```python
from build123d import *

# Parameters (mm, degrees)
SKETCH3_R           = 4.25
SKETCH3_R_2         = 3.75
BOSS_EXTRUDE1_DEPTH = 20
SKETCH21_R          = 10
BOSS_EXTRUDE2_DEPTH = 1
SKETCH29_R          = 1.75
CUT_EXTRUDE6_DEPTH  = 8.3
BOSS_EXTRUDE5_START = 1
SKETCH33_R          = 10
BOSS_EXTRUDE5_DEPTH = 1
SKETCH35_R          = 3.75
CUT_EXTRUDE8_DEPTH  = 27.153393661


with BuildPart() as part:
    # Sketch3 → Boss-Extrude1 (new body)
    with BuildSketch(Plane(origin=(0, 0, 0), x_dir=(1, 0, 0), z_dir=(0, 1, 0))):
        with Locations(Location((0, 0, 0), (0, 0, 270))):
            Circle(SKETCH3_R)
        with Locations(Location((0, 0, 0), (0, 0, 270))):
            Circle(SKETCH3_R_2, mode=Mode.SUBTRACT)
    extrude(amount=BOSS_EXTRUDE1_DEPTH)

    # Sketch21 → Boss-Extrude2 (add)
    with BuildSketch(Plane(origin=(0, 20, 0), x_dir=(1, 0, 0), z_dir=(0, 1, 0))):
        with Locations(Location((0, 0, 0), (0, 0, 270))):
            Circle(SKETCH21_R)
    extrude(amount=BOSS_EXTRUDE2_DEPTH)

    # Sketch29 → Cut-Extrude6 (cut)
    with BuildSketch(Plane(origin=(0, 21, 0), x_dir=(1, 0, 0), z_dir=(0, 1, 0))):
        with Locations(Location((0, 0, 0), (0, 0, 270))):
            Circle(SKETCH29_R)
    extrude(amount=-CUT_EXTRUDE6_DEPTH, mode=Mode.SUBTRACT)

    # Sketch33 → Boss-Extrude5 (add)
    with BuildSketch(Plane.XZ.offset(BOSS_EXTRUDE5_START)):
        with Locations(Location((0, 0, 0), (0, 0, 90))):
            Circle(SKETCH33_R)
    extrude(amount=-BOSS_EXTRUDE5_DEPTH)

    # Sketch35 → Cut-Extrude8 (cut, through all)
    with BuildSketch(Plane.XZ.offset(1)):
        with Locations(Location((0, 0, 0), (0, 0, 270))):
            Circle(SKETCH35_R)
    extrude(amount=-CUT_EXTRUDE8_DEPTH, mode=Mode.SUBTRACT)


solid = part.part
```
Read the model definition and answer for the solid it produces. Units are mm, in the model's axes. A direction names the side the tool comes from. Round coordinates to 2 decimals unless told otherwise and drop trailing zeros. Write each loop counter-clockwise with the first axis right and the second up, starting at its lowest first coordinate (ties: lowest second). Pieces come first, ordered by that corner, then holes. Notation, with made-up numbers: (16, 55.25) - (42, 55.25) arc R19 ccw to (42, 66.25) - close; hole circle Ø10 at (49, 32.25). An arc over 180 degrees is marked (long way). One line per item, written item: value.
Q1. Find section B-B (x = 2). Determine the outline of the cut face in (y, z), and give its area (3 significant figures).
The answers:
outline: (-1, -9.8) - (0, -9.8) - (0, -3.75) - (20, -3.75) - (20, -9.8) - (21, -9.8) - (21, -3.17) - (-1, -3.17) - close; (-1, 3.17) - (21, 3.17) - (21, 9.8) - (20, 9.8) - (20, 3.75) - (0, 3.75) - (0, 9.8) - (-1, 9.8) - close
area: 49.6 mm2
Q2. Each of these flat-tipped pins is pushed along its axis until it touches: P1, Ø10, axis at x = 5, y = 7.5, coming from the +Z side; P2, Ø6, axis at x = 0, z = 0, coming from the +Y side; P3, Ø1.5, axis at x = 2, y = 1.5, coming from the -Z side; P4, Ø2, axis at x = 1.5, y = 8.5, coming from the -Z side. Where does it stop, or does it pass through?
The answers:
P1: stops at z = 4.25
P2: passes through
P3: stops at z = -4.06
P4: stops at z = -4.22
Q3. Find section D-D (x = 7.75). Determine the outline of the cut face in (y, z), and give its area (3 significant figures).
The answers:
outline: (-1, -6.32) - (0, -6.32) - (0, 6.32) - (-1, 6.32) - close; (20, -6.32) - (21, -6.32) - (21, 6.32) - (20, 6.32) - close
area: 25.3 mm2
Q4. Find section A-A (z = 0). Determine the outline of the cut face in (x, y).
The answers:
outline: (-10, -1) - (-3.75, -1) - (-3.75, 21) - (-10, 21) - (-10, 20) - (-4.25, 20) - (-4.25, 0) - (-10, 0) - close; (3.75, -1) - (10, -1) - (10, 0) - (4.25, 0) - (4.25, 20) - (10, 20) - (10, 21) - (3.75, 21) - close
Q5. Find section C-C (y = 4.5). Determine the outline of the cut face in (x, z).
The answers:
outline: circle Ø8.5 at (0, 0); hole circle Ø7.5 at (0, 0)
Q6. For a pull along X with two mould halves and no side action, classify faces 1 (the flat face through (0, -1, 4)), 2 (the cylindrical face through (0.165, 9.846, 3.746)), 3 (the cylindrical face through (4.214, 9.86, -0.553)) as pulls with the +X half, pulls with the -X half, needs draft (parallel to the pull), parting line crosses it, or undercut.
The answers:
face 1: needs draft
face 2: undercut
face 3: parting line crosses it
Q7. Which of the six approach directions +Z, -Z, +X, -X, +Y, -Y give full straight-line access (tool end or side, diameter ignored) to faces 4 (the cylindrical face through (9.76, -0.51, -2.17)), 5 (the flat face through (2, 0, 4))?
The answers:
face 4: +Y, -Y
face 5: none
Q8. Straight lines are drawn through the part: line 1 (Y direction, x = -3.5, z = 7.5); line 2 (X direction, y = 9, z = 0); line 3 (X direction, y = 16.75, z = -3). For each, find the intervals that lie inside material, in ascending order. Write a range as from..to.
The answers:
line 1: y = -1..0, 20..21
line 2: x = -4.25..-3.75, 3.75..4.25
line 3: x = -3.01..-2.25, 2.25..3.01
